```python
from build123d import *

# Parameters (mm, degrees)
SKETCH1_R           = 5
BOSS_EXTRUDE1_DEPTH = 9
SKETCH2_R           = 6
BOSS_EXTRUDE2_DEPTH = 8
BOSS_EXTRUDE3_DEPTH = 5
SKETCH4_R           = 1.5
CUT_EXTRUDE1_DEPTH  = 12


with BuildPart() as part:
    # Sketch1 → Boss-Extrude1 (new body)
    with BuildSketch(Plane(origin=(0, 0, 0), x_dir=(1, 0, 0), z_dir=(0, 1, 0))):
        Circle(SKETCH1_R)
    extrude(amount=BOSS_EXTRUDE1_DEPTH)

    # Sketch2 → Boss-Extrude2 (add)
    with BuildSketch(Plane.XZ):
        Circle(SKETCH2_R)
    extrude(amount=BOSS_EXTRUDE2_DEPTH)

    # Sketch3 → Boss-Extrude3 (add)
    with BuildSketch(Plane(origin=(0, 9, 0), x_dir=(1, 0, 0), z_dir=(0, 1, 0))):
        Polygon((4.618802154, 0), (2.309401077, 4), (-2.309401077, 4), (-4.618802154, 0), (-2.309401077, -4), (2.309401077, -4), align=None)
    extrude(amount=BOSS_EXTRUDE3_DEPTH)

    # Sketch4 → Cut-Extrude1 (cut)
    with BuildSketch(Plane(origin=(0, 14, 0), x_dir=(1, 0, 0), z_dir=(0, 1, 0))):
        Circle(SKETCH4_R)
    extrude(amount=-CUT_EXTRUDE1_DEPTH, mode=Mode.SUBTRACT)


solid = part.part
```
Geometry: final body of the model. Coordinates: model frame, mm. A direction names the side the tool comes from. Give positions to 0.01 mm unless a question says otherwise; leave off trailing zeros. Loops run counter-clockwise (first coordinate to the right, second up) from the corner with the lowest first, then second, coordinate; pieces in that order, holes last. Notation, with made-up numbers: (85, 24.5) -> (93, 24.5) arc R20 cw to (93, 36.5) -> close; hole circle Ø4 at (74.25, 10). An arc over 180 degrees is marked (long way). Return JSON: item names as keys, results as strings.
Item 1: Section D-D, the plane y = 8.75. Output: boundary loops of the cut face in (x, z).
Filled in:
{"outline": "circle Ø10 at (0, 0); hole circle Ø3 at (0, 0)"}
Item 2: Section A-A, the plane x = 0. Output: boundary loops of the cut face in (y, z).
Filled in:
{"outline": "(-8, -6) -> (0, -6) -> (0, -5) -> (9, -5) -> (9, -4) -> (14, -4) -> (14, -1.5) -> (2, -1.5) -> (2, 1.5) -> (14, 1.5) -> (14, 4) -> (9, 4) -> (9, 5) -> (0, 5) -> (0, 6) -> (-8, 6) -> close"}
Item 3: Line query: line 1 (Z direction, x = 0, y = 9.25); line 2 (Z direction, x = 0, y = 6.5). Output: solid intervals per line, ascending.
Filled in:
{"line 1": "-4 to -1.5, 1.5 to 4", "line 2": "-5 to -1.5, 1.5 to 5"}
Item 4: Pin query (flat end, axial travel): P1, Ø1, axis at x = 3.5, y = 5, coming from the -Z side; P2, Ø3, axis at x = 4, y = 9.5, coming from the +Z side; P3, Ø6, axis at x = 0, y = 8, coming from the +Z side. Return the tip coordinate at first contact, or that it passes through.
Filled in:
{"P1": "z = -4", "P2": "z = 4.28", "P3": "z = 5"}
Item 5: Access query for faces 1 (the flat face through (-3.448, 11.465, -2.028)), 2 (the flat face through (3.448, 11.465, 2.028)), 3 (the flat face through (3.48, 11.46, -1.97)), 4 (the cylindrical face through (-1.08, 4.44, 4.88)), 5 (the flat face through (0, 11, -4)). Directions: +Z, -Z, +X, -X, +Y, -Y. A direction counts if a zero-diameter tool reaches every point of the face in a straight line with its end or side. Return the directions, or none.
Filled in:
{"face 1": "-Z, -X, +Y", "face 2": "+Z, +X, +Y", "face 3": "-Z, +X, +Y", "face 4": "+Y", "face 5": "-Z, +X, -X, +Y"}
Item 6: Mould query, pull axis Z, two halves, no side actions, for faces 6 (the flat face through (0, 2, 0)), 7 (the cylindrical face through (-1.5, 8.08, -0.07)), 8 (the flat face through (0, 11, 4)), 9 (the cylindrical face through (-6, -4, 0)). Classes: released by +Z, released by -Z, zero draft, split by the parting line, or undercut.
Filled in:
{"face 6": "undercut", "face 7": "undercut", "face 8": "released by +Z", "face 9": "split by the parting line"}
Item 7: Section C-C, the plane y = -4.5. Output: boundary loops of the cut face in (x, z).
Filled in:
{"outline": "circle Ø12 at (0, 0)"}
Item 8: Section B-B, the plane z = -1. Output: boundary loops of the cut face in (x, y), plus the area to 3 significant figures.
Filled in:
{"outline": "(-5.92, -8) -> (5.92, -8) -> (5.92, 0) -> (4.9, 0) -> (4.9, 9) -> (4.04, 9) -> (4.04, 14) -> (1.12, 14) -> (1.12, 2) -> (-1.12, 2) -> (-1.12, 14) -> (-4.04, 14) -> (-4.04, 9) -> (-4.9, 9) -> (-4.9, 0) -> (-5.92, 0) -> close", "area": "196 mm^2"}
